CAD build for the part. Positions are in the model's coordinates, mm. A direction names the side the tool comes from. Round coordinates to 2 decimals unless told otherwise and drop trailing zeros. Order: outer loops, then holes, each group sorted by start corner. A loop starts at its lowest first (then second) coordinate and runs counter-clockwise, first axis right, second up.
```python
from build123d import *

# Parameters (mm, degrees)
F0_W     = 406.4
F0_H     = 279.4
F1_DEPTH = 25.4
F3_DEPTH = 50.8
F5_DEPTH = 50.8
F6_W     = 38.1
F6_H     = 38.1
F7_DEPTH = 1270


with BuildPart() as f1:
    # F0 (on Front) → F1 (new body, symmetric)
    with BuildSketch(Plane.XZ):
        Polygon((-254, 25.4), (-609.6, 25.4), (-609.6, -25.4), (609.6, -25.4), (609.6, 25.4), (254, 25.4), (254, 304.8), (609.6, 304.8), (609.6, 355.6), (-609.6, 355.6), (-609.6, 304.8), (-254, 304.8), align=None)
        with Locations((0, 165.1)):
            Rectangle(F0_W, F0_H, mode=Mode.SUBTRACT)
    extrude(amount=F1_DEPTH, both=True)

    # F2 (on face) → F3 (join)
    with BuildSketch(Plane.XY.offset(355.6)):
        Polygon((-609.6, 76.2), (-609.6, 25.4), (-603.25, 25.4), (-558.8, 25.4), (-558.8, 31.75), (-603.25, 31.75), (-603.25, 76.2), align=None)
        Polygon((-609.6, -25.4), (-609.6, -76.2), (-603.25, -76.2), (-603.25, -31.75), (-558.8, -31.75), (-558.8, -25.4), (-603.25, -25.4), align=None)
        Polygon((603.25, -25.4), (558.8, -25.4), (558.8, -31.75), (603.25, -31.75), (603.25, -76.2), (609.6, -76.2), (609.6, -25.4), align=None)
        Polygon((603.25, 25.4), (609.6, 25.4), (609.6, 76.2), (603.25, 76.2), (603.25, 31.75), (558.8, 31.75), (558.8, 25.4), align=None)
    extrude(amount=-F3_DEPTH)

    # F4 (on face) → F5 (join)
    with BuildSketch(Plane(origin=(0, 0, -25.4), x_dir=(1, 0, 0), z_dir=(0, 0, -1))):
        Polygon((-603.25, -76.2), (-603.25, -31.75), (-558.8, -31.75), (-558.8, -25.4), (-603.25, -25.4), (-609.6, -25.4), (-609.6, -76.2), align=None)
        Polygon((-558.8, 31.75), (-603.25, 31.75), (-603.25, 76.2), (-609.6, 76.2), (-609.6, 25.4), (-603.25, 25.4), (-558.8, 25.4), align=None)
        Polygon((558.8, 25.4), (603.25, 25.4), (609.6, 25.4), (609.6, 76.2), (603.25, 76.2), (603.25, 31.75), (558.8, 31.75), align=None)
        Polygon((558.8, -31.75), (603.25, -31.75), (603.25, -76.2), (609.6, -76.2), (609.6, -25.4), (603.25, -25.4), (558.8, -25.4), align=None)
    extrude(amount=-F5_DEPTH)

    # F6 (on Right) → F7 (cut, symmetric)
    with BuildSketch(Plane.YZ):
        with Locations((0, 330.2)):
            Rectangle(F6_W, F6_H)
        Rectangle(F6_W, F6_H)
    extrude(amount=F7_DEPTH, both=True, mode=Mode.SUBTRACT)


solid = f1.part
```
1. Cut at A-A, the plane y = -5. Write the cut outline in (x, z).
2. Mould opens along X. For faces 6 (the face through (-581, -31.75, 331)), 7 (the face through (254, 0, 163)), 8 (the face through (446, -6, 25.4)) say: released by +X, released by -X, zero draft, split by the parting line, or undercut.
3. Drill centre lines: line 1 (Z direction, x = -171, y = -8.5); line 2 (X direction, y = 30.5, z = 311); line 3 (X direction, y = -1, z = 30). Where is each one in solid material? Low to high.
4. Cut at D-D, the plane y = 58.5. Write the cut outline in (x, z).
5. Cut at C-C, the plane x = 91. Write the cut outline in (y, z), and give its area (3 significant figures).
6. Pin check, flat tips, straight feed: P1, Ø1.5, axis at x = -220.5, z = 80, coming from the +Y side; P2, Ø13.5, axis at x = -572, z = 341.5, coming from the -Y side; P3, Ø15, axis at y = 10.5, z = 179.5, coming from the -X side. Stop position of each tip, or through.
7. Tool access for faces 1 (the face through (-446, -6, 25.4)), 2 (the face through (581, -31.75, 331)), 3 (the face through (-603.25, 54, 331)), 4 (the face through (9, 19.05, 0)), 5 (the face through (-203.2, 0, 163)): list every direction of +Z, -Z, +X, -X, +Y, -Y with a clear straight run to the whole face (end or side of a thin tool).
8. Cut at B-B, the plane z = 41. Write the cut outline in (x, y), and give its area (3 significant figures).
Outcome:
1. outline: (-609.6, -25.4) - (609.6, -25.4) - (609.6, -19.05) - (-609.6, -19.05) - close; (-609.6, 19.05) - (609.6, 19.05) - (609.6, 25.4) - (254, 25.4) - (254, 304.8) - (609.6, 304.8) - (609.6, 311.15) - (-609.6, 311.15) - (-609.6, 304.8) - (-254, 304.8) - (-254, 25.4) - (-609.6, 25.4) - close; (-609.6, 349.25) - (609.6, 349.25) - (609.6, 355.6) - (-609.6, 355.6) - close; hole (-203.2, 25.4) - (203.2, 25.4) - (203.2, 304.8) - (-203.2, 304.8) - close
2. face 6: undercut
2. face 7: released by +X
2. face 8: zero draft
3. line 1: z = -25.4 to -19.05, 19.05 to 25.4, 304.8 to 311.15, 349.25 to 355.6
3. line 2: x = -609.6 to -558.8, 558.8 to 609.6
3. line 3: x = -254 to -203.2, 203.2 to 254
4. outline: (-609.6, -25.4) - (-603.25, -25.4) - (-603.25, 25.4) - (-609.6, 25.4) - close; (-609.6, 304.8) - (-603.25, 304.8) - (-603.25, 355.6) - (-609.6, 355.6) - close; (603.25, -25.4) - (609.6, -25.4) - (609.6, 25.4) - (603.25, 25.4) - close; (603.25, 304.8) - (609.6, 304.8) - (609.6, 355.6) - (603.25, 355.6) - close
5. outline: (-25.4, -25.4) - (25.4, -25.4) - (25.4, 25.4) - (-25.4, 25.4) - close; (-25.4, 304.8) - (25.4, 304.8) - (25.4, 355.6) - (-25.4, 355.6) - close; hole (-19.05, -19.05) - (19.05, -19.05) - (19.05, 19.05) - (-19.05, 19.05) - close; hole (-19.05, 311.15) - (19.05, 311.15) - (19.05, 349.25) - (-19.05, 349.25) - close
5. area: 2,260 mm2
6. P1: stops at y = 25.4
6. P2: stops at y = -31.75
6. P3: stops at x = -254
7. face 1: -X, +Y, -Y
7. face 2: +Z, -Z, -Y
7. face 3: +Z, -Z, +Y
7. face 4: +X, -X
7. face 5: +Y, -Y
8. outline: (-254, -25.4) - (-203.2, -25.4) - (-203.2, 25.4) - (-254, 25.4) - close; (203.2, -25.4) - (254, -25.4) - (254, 25.4) - (203.2, 25.4) - close
8. area: 5,160 mm2
